Check sheet for the modelled part. Datum: model origin and axes. Units: mm. A direction names the side the tool comes from. Coordinates: 2 decimals unless noted, no trailing zeros. Write each loop counter-clockwise with the first axis right and the second up, starting at its lowest first coordinate (ties: lowest second). Pieces come first, ordered by that corner, then holes. Notation, with made-up numbers: (77, -24.75) - (131, -24.75) arc R28 ccw to (131, 1.25) - close; hole circle Ø9 at (15, 16.25). An arc over 180 degrees is marked (long way). Write each question's results on one line, items separated by ' | '.
from build123d import *

# Parameters (mm, degrees)
SKETCH2_W                 = 18.5
SKETCH2_H                 = 25.41
BOSS_EXTRUDE1_DEPTH       = 9
CUT_EXTRUDE1_DEPTH        = 25.41
F_0_80_TAPPED_HOLE1_D     = 1.19126
F_0_80_TAPPED_HOLE1_DEPTH = 3.642109389
F_0_80_TAPPED_HOLE1_TIP   = 0.357890611
CUT_EXTRUDE3_DEPTH        = 33.694312961
CUT_EXTRUDE3_DEPTH_BACK   = 25.41
F_2_56_TAPPED_HOLE3_D     = 1.778
F_2_56_TAPPED_HOLE3_DEPTH = 3.46583491
F_2_56_TAPPED_HOLE3_TIP   = 0.53416509


with BuildPart() as part:
    # Sketch2 → Boss-Extrude1 (new body)
    with BuildSketch(Plane(origin=(0, 0, 0), x_dir=(1, 0, 0), z_dir=(0, 1, 0))):
        with Locations((9.25, 12.705)):
            Rectangle(SKETCH2_W, SKETCH2_H)
    extrude(amount=BOSS_EXTRUDE1_DEPTH)

    # Sketch6 → Cut-Extrude1 (cut)
    with BuildSketch(Plane.XY):
        with BuildLine():
            Line((2.9, 9), (15.6, 9))
            ThreePointArc((15.6, 9), (9.25, 2.65), (2.9, 9))
        make_face()
    extrude(amount=-CUT_EXTRUDE1_DEPTH, mode=Mode.SUBTRACT)

    # #0-80 Tapped Hole1
    with Locations(Plane(origin=(0, 9, 0), x_dir=(1, 0, 0), z_dir=(0, 1, 0))):
        with Locations((17.05, 20.41), (17.05, 5)):
            Hole(F_0_80_TAPPED_HOLE1_D / 2, depth=F_0_80_TAPPED_HOLE1_DEPTH)
            with Locations((0, 0, -(F_0_80_TAPPED_HOLE1_DEPTH + F_0_80_TAPPED_HOLE1_TIP / 2))):  # 118° drill point
                Cone(0, F_0_80_TAPPED_HOLE1_D / 2, F_0_80_TAPPED_HOLE1_TIP, mode=Mode.SUBTRACT)

    # Sketch14 → Cut-Extrude3 (cut, two sides)
    with BuildSketch(Plane(origin=(0, 0, -25.41), x_dir=(-1, 0, 0), z_dir=(0, 0, -1))) as cut_extrude3_sk:
        Polygon((0, 60.146081223), (0, 9), (0, 7.5), (-3.246658661, 7.5), (-2.9, 9), (8.616604878, 58.832614185), (24.031387378, 159.956651774), (15.4147825, 161.270118812), align=None)
    extrude(amount=CUT_EXTRUDE3_DEPTH, mode=Mode.SUBTRACT)
    extrude(cut_extrude3_sk.sketch, amount=-CUT_EXTRUDE3_DEPTH_BACK, mode=Mode.SUBTRACT)


with BuildPart() as cut_extrude3_kept_piece:
    # of the separate pieces the step leaves, the one the design keeps (cut_extrude3_pieces_kept)
    add(part.part.solids().sort_by_distance((0, 0, 0))[0])

    # #2-56 Tapped Hole3
    with Locations(Plane(origin=(0, 0, 0), x_dir=(-1, 0, 0), z_dir=(0, -1, 0))):
        with Locations((-17, 12.705), (-1.5, 12.705)):
            Hole(F_2_56_TAPPED_HOLE3_D / 2, depth=F_2_56_TAPPED_HOLE3_DEPTH)
            with Locations((0, 0, -(F_2_56_TAPPED_HOLE3_DEPTH + F_2_56_TAPPED_HOLE3_TIP / 2))):  # 118° drill point
                Cone(0, F_2_56_TAPPED_HOLE3_D / 2, F_2_56_TAPPED_HOLE3_TIP, mode=Mode.SUBTRACT)


solid = cut_extrude3_kept_piece.part
1. Material ranges on L1, parallel to Z at x = 17.05, y = 6.3; L2, parallel to Z at x = 1.5, y = 2.5; L3, parallel to X at y = 7, z = -12.75, recorded low to high. Write a range as [from, to].
Values follow:
L1: z = [-25.41, -21.01], [-19.81, -5.6], [-4.4, 0] | L2: z = [-25.41, -13.59], [-11.82, 0] | L3: x = [0, 3.22], [15.28, 18.5]
2. Sectioned sample at A-A (z = -7.5). Record the cut outline in (x, y), then the cut area to 3 significant figures.
Values follow:
outline: (0, 0) - (18.5, 0) - (18.5, 9) - (15.6, 9) arc R6.35 cw to (3.08, 7.5) - (0, 7.5) - close | area: 98.7 mm^2
3. Draft check along Z on faces 6 (the conical face through (1.62, 3.91, -12.61)), 7 (the flat face through (0, 4, -13)), 8 (the conical face through (16.974, 5.062, -5.07)), 9 (the flat face through (9, 2, -25.41)). Enter one of: pulls with the +Z half, pulls with the -Z half, needs draft (parallel to the pull), parting line crosses it, or undercut.
Values follow:
face 6: undercut | face 7: needs draft | face 8: undercut | face 9: pulls with the -Z half
4. Go/stop test with flat-tipped pins: pin 1 (3.5 mm diameter, centred on x = 1.5, z = -15.5, fed in from +Y); pin 2 (1.1 mm diameter, centred on x = 1.5, z = -12.705, fed in from -Y); pin 3 (3 mm diameter, centred on x = 6, z = -15, fed in from +Y). Record where each tip stops, or that it passes through.
Values follow:
pin 1: stops at y = 7.5 | pin 2: stops at y = 3.67 | pin 3: stops at y = 4.79
5. Sectioned sample at B-B (y = 4.5). Record the cut outline in (x, z).
Values follow:
outline: (0, -25.41) - (4.77, -25.41) - (4.77, 0) - (0, 0) - close; (13.73, -25.41) - (18.5, -25.41) - (18.5, 0) - (13.73, 0) - close
6. Sectioned sample at D-D (x = 6). Record the cut outline in (y, z).
Values follow:
outline: (0, -25.41) - (3.54, -25.41) - (3.54, 0) - (0, 0) - close
7. Sectioned sample at C-C (x = 13). Record the cut outline in (y, z).
Values follow:
outline: (0, -25.41) - (3.88, -25.41) - (3.88, 0) - (0, 0) - close
8. Access from +Z, -Z, +X, -X, +Y, -Y to the whole of each face (thin tool, end or side, straight path). Record for faces 1 (the flat face through (2, 7.5, -13)), 2 (the cylindrical face through (10.13, 2.71, -12.53)), 3 (the cylindrical face through (17.13, 7.15, -5.59)), 4 (the flat face through (17, 9, -13)), 5 (the cylindrical face through (1.91, 1.757, -11.916)).
Values follow:
face 1: +Z, -Z, -X, +Y | face 2: +Z, -Z, +Y | face 3: +Y | face 4: +Z, -Z, +X, -X, +Y | face 5: -Y
